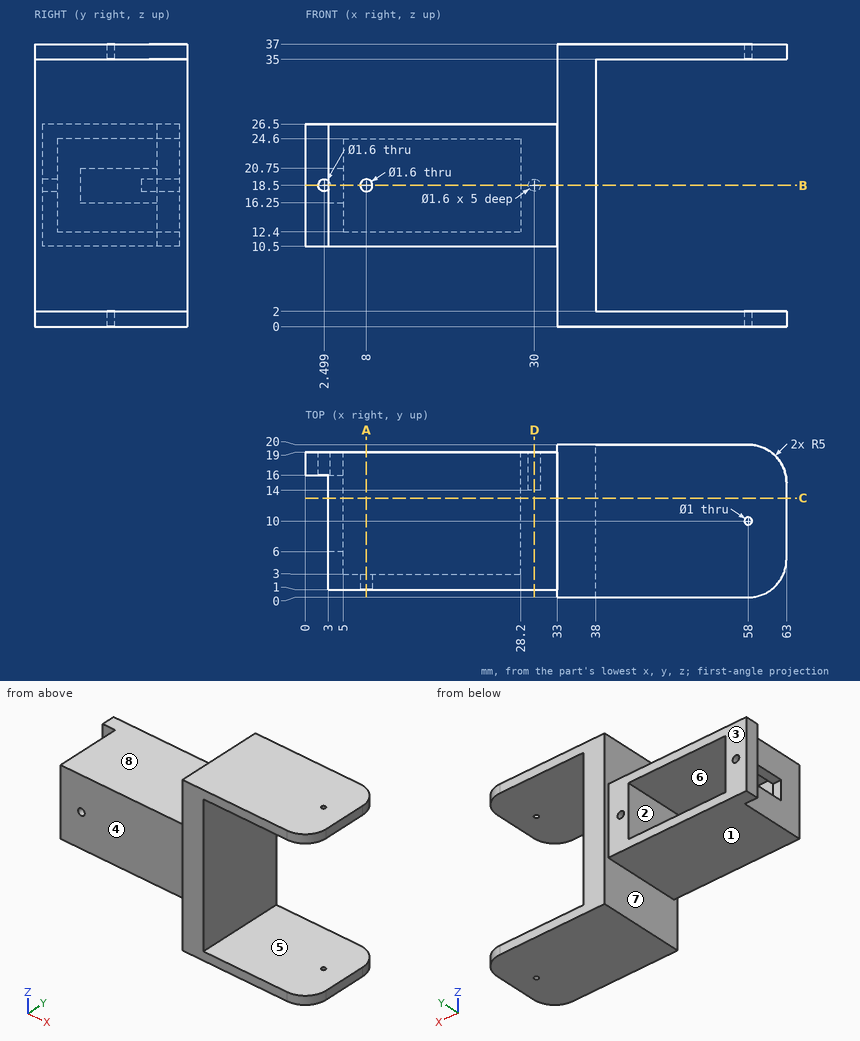
Can you work these out from the drawing? Everything is in mm from the part's minimum corner. A direction names the side the tool comes from. Give positions to 0.01 mm unless a question says otherwise; leave off trailing zeros. Loops run counter-clockwise (first coordinate to the right, second up) from the corner with the lowest first, then second, coordinate; pieces in that order, holes last. Notation, with made-up numbers: (5.5, -4) -> (21.5, -4) arc R14 ccw to (21.5, 6) -> close; hole circle Ø5 at (3, 58). An arc over 180 degrees is marked (long way). Return JSON: item names as keys, results as strings.
Q1. On a 3-axis mill with a long thin cutter (end or side, diameter ignored), from which of +Z, -Z, +X, -X, +Y, -Y can I reach the whole of each face in a straight line? I mean the marked faces 1, 2, 3, 4 and 5. Say none if no direction works.
Checks:
{"face 1": "-Z, -X, +Y, -Y", "face 2": "+Y", "face 3": "+Z, -Z, -X, +Y", "face 4": "+Z, -Z, -X, -Y", "face 5": "+X, +Y, -Y"}
Q2. I need wall thicknesses on probe 1 along Z at (x, y) = (49, 13); probe 2 along X at (y, z) = (10, 36.6); probe 3 along X at (y, z) = (5.75, 17.5). Which ranges of each line are inside material? Lowest first, please.
Checks:
{"probe 1": "z = 0 to 2, 35 to 37", "probe 2": "x = 33 to 57.5, 58.5 to 63", "probe 3": "x = 3 to 5, 28.2 to 38"}
Q3. I want a section at C-C, the plane y = 13. List the corners of the cut face in (x, z) for me.
Checks:
{"outline": "(3, 10.5) -> (33, 10.5) -> (33, 0) -> (63, 0) -> (63, 2) -> (38, 2) -> (38, 35) -> (63, 35) -> (63, 37) -> (33, 37) -> (33, 26.5) -> (3, 26.5) -> (3, 20.75) -> (5, 20.75) -> (5, 24.6) -> (28.2, 24.6) -> (28.2, 12.4) -> (5, 12.4) -> (5, 16.25) -> (3, 16.25) -> close"}
Q4. We'd pull the mould along Z, two halves only. Please class the marked faces 6, 7 and 8: released by +Z, released by -Z, zero draft, split by the parting line, or undercut.
Checks:
{"face 6": "undercut", "face 7": "zero draft", "face 8": "released by +Z"}
Q5. I want a section at B-B, the plane z = 18.5. List the corners of the cut face in (x, y) for me, then the cut area to 3 significant figures.
Checks:
{"outline": "(0, 16) -> (1.7, 16) -> (1.7, 19) -> (0, 19) -> close; (3, 1) -> (7.2, 1) -> (7.2, 3) -> (5, 3) -> (5, 6) -> (3, 6) -> close; (3.3, 16) -> (5, 16) -> (5, 19) -> (3.3, 19) -> close; (8.8, 1) -> (33, 1) -> (33, 0) -> (38, 0) -> (38, 20) -> (33, 20) -> (33, 19) -> (30.8, 19) -> (30.8, 14) -> (29.2, 14) -> (29.2, 19) -> (28.2, 19) -> (28.2, 3) -> (8.8, 3) -> close", "area": "242 mm2"}
Q6. I want a section at A-A, the plane x = 8. List the corners of the cut face in (y, z) for me.
Checks:
{"outline": "(1, 10.5) -> (19, 10.5) -> (19, 12.4) -> (3, 12.4) -> (3, 17.7) -> (1, 17.7) -> close; (1, 19.3) -> (3, 19.3) -> (3, 24.6) -> (19, 24.6) -> (19, 26.5) -> (1, 26.5) -> close"}
Q7. For pin 1 Ø1.3 at (x, z) = (2.5, 18.5) entering from +Y; pin 2 Ø0.6 at (x, y) = (3.5, 13) entering from +Z; pin 3 Ø10 at (y, z) = (11.5, 19) entering from -X; pin 4 Ø3 at (y, z) = (10.5, 32) entering from -X, each with a flat end and sliding along its axis, tell me the tip position at first contact or that it passes through.
Checks:
{"pin 1": "stops at y = 6", "pin 2": "stops at z = 26.5", "pin 3": "stops at x = 0", "pin 4": "stops at x = 33"}
Q8. I want a section at D-D, the plane x = 30. List the corners of the cut face in (y, z) for me, then the cut area to 3 significant figures.
Checks:
{"outline": "(1, 10.5) -> (19, 10.5) -> (19, 17.7) -> (14, 17.7) -> (14, 19.3) -> (19, 19.3) -> (19, 26.5) -> (1, 26.5) -> close", "area": "280 mm2"}
